Source: CAD feature listing. Evaluate the final solid. Frame: model axes, mm. Face numbers are marked on the shaded views. A direction names the side the tool comes from. Coordinates: 2 decimals unless noted, no trailing zeros. Loops run counter-clockwise (first coordinate to the right, second up) from the corner with the lowest first, then second, coordinate; pieces in that order, holes last. Notation, with made-up numbers: (40.5, -3) - (51.5, -3) arc R30 ccw to (51.5, 32) - close; hole circle Ø10 at (89.5, -6.75). An arc over 180 degrees is marked (long way). Write item = value, one per line. Start each with the question number.
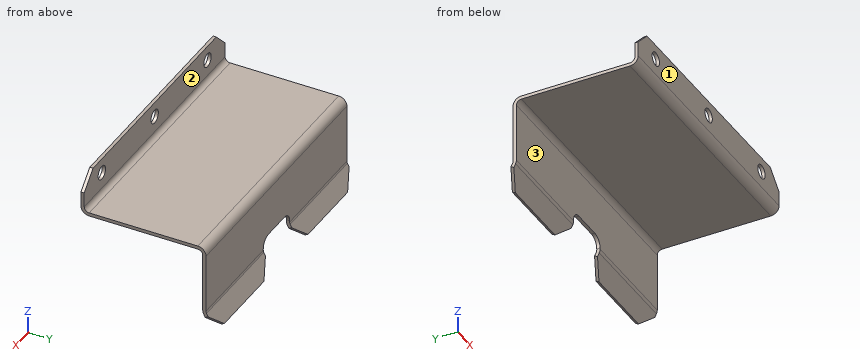
from build123d import *

# Parameters (mm, degrees)
BASE_FLANGE1_DEPTH       = 80
SKETCH7_R                = 2.1
CUT_EXTRUDE2_DEPTH       = 94.099760047
LPATTERN1_COUNT          = 2
LPATTERN1_PITCH          = 30
LPATTERN1_COL_COUNT      = 2
LPATTERN1_COL_PITCH      = 30
CUT_EXTRUDE_1_DEPTH      = 93.303846074
CUT_EXTRUDE_1_DEPTH_BACK = 93.303846074
SKETCH_1_W               = 15
SKETCH_1_H               = 10
CHAMFER_1_SIZE           = 5
FILLET_1_R               = 3


# Read off the part's stored shape, not the designer's step: Base-Flange1
with BuildPart() as part:
    # Base-Flange1 outline → Base-Flange1 (new body)
    with BuildSketch(Plane(origin=(0, 0, 0), x_dir=(0, 0, -1), z_dir=(1, 0, 0))):
        with BuildLine():
            Line((-2.5, -17.5), (-12, -17.5))
            Line((-12, -17.5), (-12, -18.5))
            Line((-12, -18.5), (-2.5, -18.5))
            ThreePointArc((-2.5, -18.5), (-0.732233047, -17.767766953), (0, -16))
            Line((0, -16), (0, 17))
            ThreePointArc((0, 17), (0.439339828, 18.060660172), (1.5, 18.5))
            Line((1.5, 18.5), (19.409830056, 18.5))
            ThreePointArc((19.409830056, 18.5), (19.984212358, 18.566877526), (20.527864045, 18.763932023))
            Line((20.527864045, 18.763932023), (26, 21.5))
            Line((26, 21.5), (25.552786405, 22.394427191))
            Line((25.552786405, 22.394427191), (20.08065045, 19.658359214))
            ThreePointArc((20.08065045, 19.658359214), (19.754459437, 19.540126516), (19.409830056, 19.5))
            Line((19.409830056, 19.5), (1.5, 19.5))
            ThreePointArc((1.5, 19.5), (-0.267766953, 18.767766953), (-1, 17))
            Line((-1, 17), (-1, -16))
            ThreePointArc((-1, -16), (-1.439339828, -17.060660172), (-2.5, -17.5))
        make_face()
    extrude(amount=BASE_FLANGE1_DEPTH)

    # Sketch7 → Cut-Extrude2 (cut, through all)
    with BuildSketch(Plane(origin=(0, -17.5, 0), x_dir=(1, 0, 0), z_dir=(0, 1, 0))):
        with Locations(Location((40, -7.5, 0), (0, 0, 270))):
            Circle(SKETCH7_R)
    cut_extrude2 = extrude(amount=-CUT_EXTRUDE2_DEPTH, mode=Mode.SUBTRACT)

    # LPattern1: Cut-Extrude2 ×2
    with Locations(*[(i * LPATTERN1_PITCH, 0, 0) for i in range(1, LPATTERN1_COUNT)]):
        add(cut_extrude2, mode=Mode.SUBTRACT)

    # LPattern1 col: Cut-Extrude2 ×2
    with Locations(*[(-i * LPATTERN1_COL_PITCH, 0, 0) for i in range(1, LPATTERN1_COL_COUNT)]):
        add(cut_extrude2, mode=Mode.SUBTRACT)

    # Sketch 1 → 除料-伸長1 (cut, two sides: drawn at the far end of the back side and taken through both)
    with BuildSketch(Plane(origin=(0, 19.5, 0), x_dir=(1, 0, 0), z_dir=(0, 1, 0)).offset(-CUT_EXTRUDE_1_DEPTH_BACK)):
        with Locations((40, 21)):
            Rectangle(SKETCH_1_W, SKETCH_1_H)
    extrude(amount=CUT_EXTRUDE_1_DEPTH + CUT_EXTRUDE_1_DEPTH_BACK, mode=Mode.SUBTRACT)

    # 導角1
    chamfer_1_edges = [part.edges().sort_by_distance(p)[0] for p in [
        (32.5, 21.947213595, -25.776393202),
        (47.5, 21.947213595, -25.776393202),
        (0, 21.947213595, -25.776393202),
        (0, -18, 12),
        (80, 21.947213595, -25.776393202),
        (80, -18, 12),
    ]]
    chamfer(chamfer_1_edges, length=CHAMFER_1_SIZE)

    # 圓角1
    fillet_1_edges = [part.edges().sort_by_distance(p)[0] for p in [
        (32.5, 19, -16),
        (47.5, 19, -16),
    ]]
    fillet(fillet_1_edges, radius=FILLET_1_R)


solid = part.part
Item 1: Cut plane A-A (x = 10). Return the cut outline in (y, z), then the cut area to 3 significant figures.
Item 2: Cut plane C-C (x = 40). Return the cut outline in (y, z), then the cut area to 3 significant figures.
Item 3: Cut plane B-B (z = -17). Return the cut outline in (x, y), then the cut area to 3 significant figures.
Item 4: Cut plane D-D (x = 60.5). Return the cut outline in (y, z).
Item 5: First-contact query: pin 1 (2 mm diameter, centred on x = 24, y = -9, fed in from -Z); pin 2 (10.5 mm diameter, centred on x = 28.5, z = 9.5, fed in from +Y); pin 3 (2 mm diameter, centred on x = 65, z = -8.5, fed in from -Y). Flat tips, straight axial feed; report the tip coordinate or a pass-through.
Item 6: Reachability of the marked faces 1, 2 and 3 from +Z, -Z, +X, -X, +Y, -Y: full face, straight path, thin tool, end or side. Return the list, or none.
Item 7: Material intervals for L1, parallel to X at y = -18, z = 7; L2, parallel to X at y = -17.65, z = 7.5; L3, parallel to Y at x = 69, z = -15.5, sorted ascending. Write a range as [from, to].
Responses:
q1.outline = (-18.5, 2.5) arc R2.5 ccw to (-16, 0) - (17, 0) arc R1.5 cw to (18.5, -1.5) - (18.5, -19.41) arc R2.5 ccw to (18.76, -20.53) - (21.5, -26) - (22.39, -25.55) - (19.66, -20.08) arc R1.5 cw to (19.5, -19.41) - (19.5, -1.5) arc R2.5 ccw to (17, 1) - (-16, 1) arc R1.5 cw to (-17.5, 2.5) - (-17.5, 5.4) - (-18.5, 5.4) - close; (-18.5, 9.6) - (-17.5, 9.6) - (-17.5, 12) - (-18.5, 12) - close
q1.area = 69.5 mm2
q2.outline = (-18.5, 2.5) arc R2.5 ccw to (-16, 0) - (17, 0) arc R1.5 cw to (18.5, -1.5) - (18.5, -16) - (19.5, -16) - (19.5, -1.5) arc R2.5 ccw to (17, 1) - (-16, 1) arc R1.5 cw to (-17.5, 2.5) - (-17.5, 5.4) - (-18.5, 5.4) - close; (-18.5, 9.6) - (-17.5, 9.6) - (-17.5, 12) - (-18.5, 12) - close
q2.area = 59.1 mm2
q3.outline = (0, 18.5) - (33.26, 18.5) - (33.26, 19.5) - (0, 19.5) - close; (46.74, 18.5) - (80, 18.5) - (80, 19.5) - (46.74, 19.5) - close
q3.area = 66.5 mm2
q4.outline = (-18.5, 2.5) arc R2.5 ccw to (-16, 0) - (17, 0) arc R1.5 cw to (18.5, -1.5) - (18.5, -19.41) arc R2.5 ccw to (18.76, -20.53) - (21.5, -26) - (22.39, -25.55) - (19.66, -20.08) arc R1.5 cw to (19.5, -19.41) - (19.5, -1.5) arc R2.5 ccw to (17, 1) - (-16, 1) arc R1.5 cw to (-17.5, 2.5) - (-17.5, 12) - (-18.5, 12) - close
q5.pin_1 = 0
q5.pin_2 = -17.5
q5.pin_3 = 18.5
q6.face_1 = +Z, -Z, +X, -X, -Y
q6.face_2 = +Z, +X, -X, +Y
q6.face_3 = -Z, +X, -X, -Y
q7.L1 = [0, 7.96], [12.04, 37.96], [42.04, 67.96], [72.04, 80]
q7.L2 = [0.5, 7.9], [12.1, 37.9], [42.1, 67.9], [72.1, 79.5]
q7.L3 = [18.5, 19.5]
